Input: part model. Units: mm. Frame: model coordinates. Face numbers are marked on the shaded views. A direction names the side the tool comes from. Coordinates: 2 decimals unless noted, no trailing zeros. Write each loop counter-clockwise with the first axis right and the second up, starting at its lowest first coordinate (ties: lowest second). Pieces come first, ordered by that corner, then holes. Notation, with made-up numbers: (41, 68.5) - (62, 68.5) arc R23 ccw to (62, 107.5) - close; hole circle Ø11 at (62, -6.75). An arc over 180 degrees is marked (long way). Use a Markdown table: item, result. Add a question column.
Q1. Mould query, pull axis Y, two halves, no side actions, for the marked faces 1, 2 and 3. Classes: released by +Y, released by -Y, zero draft, split by the parting line, or undercut.
Q2. Section query A-A (x = 0). Return the cut outline in (y, z).
Q3. Pin query (flat end, axial travel): P1, Ø4, axis at y = 0.5, z = 5.5, coming from the +X side; P2, Ø9, axis at x = 0, y = 0, coming from the -Z side; P3, Ø4, axis at x = -6, z = 1.5, coming from the -Y side; P4, Ø1.5, axis at x = -6.5, y = 5.5, coming from the +Z side. Return the tip coordinate at first contact, or that it passes through.
Q4. Section query C-C (z = 10). Return the cut outline in (x, y).
Q5. Section query D-D (y = -7.25). Return the cut outline in (x, z).
Q6. Material intervals for probe 1 along Y at (x, z) = (0, 8.5); probe 2 along Y at (x, z) = (0, 1.2); probe 3 along Z at (x, y) = (-2.25, 4), sorted ascending. Write a range as from..to.
Q7. Set-up query: the marked faces 4, 5 and 6. Return all of +Z, -Z, +X, -X, +Y, -Y with unobstructed straight access to the full face (end or side cutting, diameter ignored); none if empty.
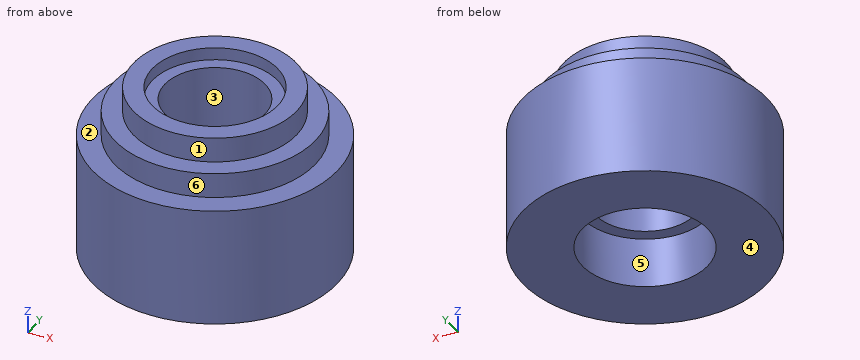
from build123d import *

# Parameters (mm, degrees)
SKETCH_1_R          = 9.75
EXTRUDE_1_DEPTH     = 9.5
SKETCH_2_R          = 8
EXTRUDE_2_DEPTH     = 2
SKETCH_3_R          = 6.5
EXTRUDE_3_DEPTH     = 2
SKETCH_4_R          = 4
CUT_EXTRUDE_1_DEPTH = 20.297020495
SKETCH_5_R          = 5
CUT_EXTRUDE_2_DEPTH = 4
CUT_EXTRUDE_START   = -1
SKETCH_6_R          = 5
CUT_EXTRUDE_3_DEPTH = 1


with BuildPart() as part:
    # 스케치1 → 돌출1 (new body)
    with BuildSketch(Plane.XY):
        Circle(SKETCH_1_R)
    extrude(amount=EXTRUDE_1_DEPTH)

    # 스케치2 → 돌출2 (add)
    with BuildSketch(Plane.XY.offset(9.5)):
        Circle(SKETCH_2_R)
    extrude(amount=EXTRUDE_2_DEPTH)

    # 스케치3 → 돌출3 (add)
    with BuildSketch(Plane.XY.offset(11.5)):
        Circle(SKETCH_3_R)
    extrude(amount=EXTRUDE_3_DEPTH)

    # 스케치4 → 컷-돌출1 (cut, through all)
    with BuildSketch(Plane(origin=(0, 0, 0), x_dir=(-1, 0, 0), z_dir=(0, 0, -1))):
        Circle(SKETCH_4_R)
    extrude(amount=-CUT_EXTRUDE_1_DEPTH, mode=Mode.SUBTRACT)

    # 스케치5 → 컷-돌출2 (cut)
    with BuildSketch(Plane(origin=(0, 0, 0), x_dir=(-1, 0, 0), z_dir=(0, 0, -1))):
        Circle(SKETCH_5_R)
    extrude(amount=-CUT_EXTRUDE_2_DEPTH, mode=Mode.SUBTRACT)

    # 스케치6 → 컷-돌출3 (cut)
    with BuildSketch(Plane.XY.offset(13.5).offset(CUT_EXTRUDE_START)):
        with Locations(Location((0, 0, 0), (0, 0, 180))):
            Circle(SKETCH_6_R)
    extrude(amount=CUT_EXTRUDE_3_DEPTH, mode=Mode.SUBTRACT)


solid = part.part
Values follow:
| question | item | result |
|---|---|---|
| 1 | face 1 | split by the parting line |
| 1 | face 2 | zero draft |
| 1 | face 3 | undercut |
| 2 | outline | (-9.75, 0) - (-5, 0) - (-5, 4) - (-4, 4) - (-4, 12.5) - (-5, 12.5) - (-5, 13.5) - (-6.5, 13.5) - (-6.5, 11.5) - (-8, 11.5) - (-8, 9.5) - (-9.75, 9.5) - close; (4, 4) - (5, 4) - (5, 0) - (9.75, 0) - (9.75, 9.5) - (8, 9.5) - (8, 11.5) - (6.5, 11.5) - (6.5, 13.5) - (5, 13.5) - (5, 12.5) - (4, 12.5) - close |
| 3 | P1 | x = 9.75 |
| 3 | P2 | z = 4 |
| 3 | P3 | y = -8.89 |
| 3 | P4 | z = 11.5 |
| 4 | outline | circle Ø16 at (0, 0); hole circle Ø8 at (0, 0) |
| 5 | outline | (-6.52, 0) - (6.52, 0) - (6.52, 9.5) - (3.38, 9.5) - (3.38, 11.5) - (-3.38, 11.5) - (-3.38, 9.5) - (-6.52, 9.5) - close |
| 6 | probe 1 | -9.75..-4, 4..9.75 |
| 6 | probe 2 | -9.75..-5, 5..9.75 |
| 6 | probe 3 | 4..12.5 |
| 7 | face 4 | -Z, +X, -X, +Y, -Y |
| 7 | face 5 | -Z |
| 7 | face 6 | +Z |
